Check sheet for the drawn part. Datum: minimum x, y, z corner. Units: mm. A direction names the side the tool comes from. Give positions to 0.01 mm unless a question says otherwise; leave off trailing zeros. Loops run counter-clockwise (first coordinate to the right, second up) from the corner with the lowest first, then second, coordinate; pieces in that order, holes last. Notation, with made-up numbers: (-28, 69.5) - (-22, 69.5) arc R26 ccw to (-22, 97.5) - close; hole circle Ø11 at (-34.75, 83.5). An arc over 180 degrees is marked (long way). Use one line per item in the form item = value.
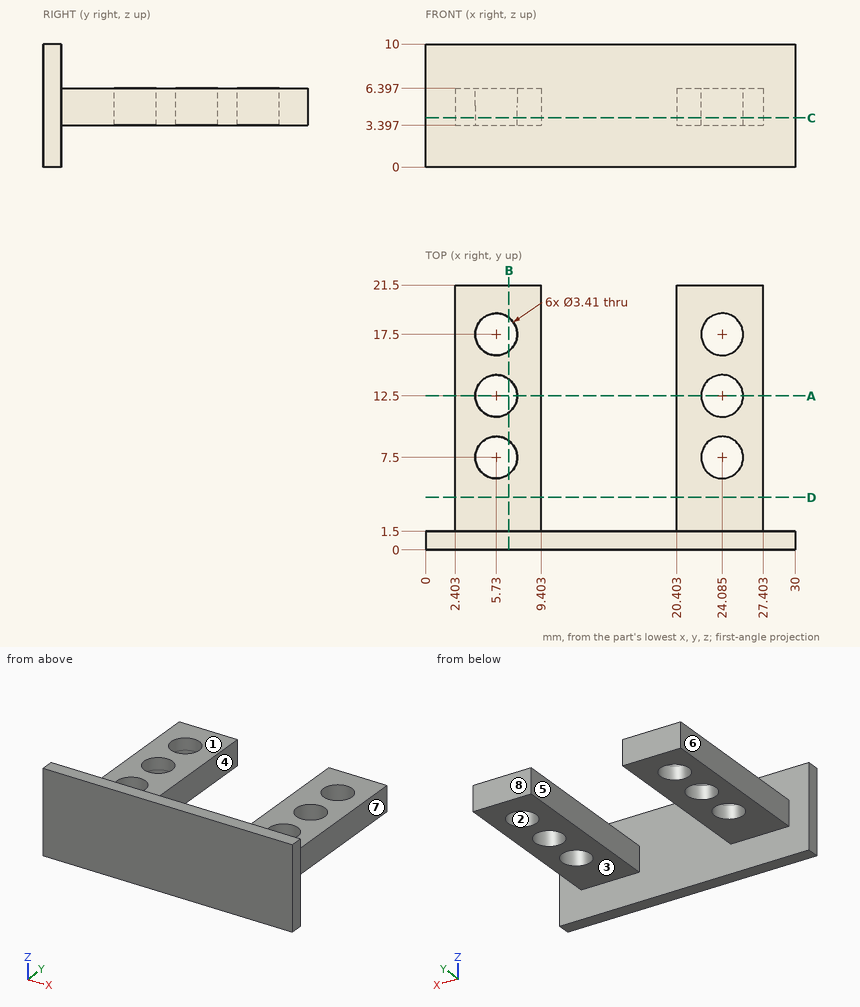
1. Scan lines: probe 1 along X at (y, z) = (12.5, 5.55) (1 decimal); probe 2 along X at (y, z) = (10.5, 4); probe 3 along Y at (x, z) = (10.25, 3.5). Record each from-to range of solid material in increasing order.
Result set:
probe_1 = 2.4 to 4, 7.4 to 9.4, 20.4 to 22.4, 25.8 to 27.4
probe_2 = 2.4 to 9.4, 20.4 to 27.4
probe_3 = 0 to 1.5
2. Section check D-D, the plane y = 4.25. Record the cut outline in (x, z), then the cut area to 3 significant figures.
Result set:
outline = (2.4, 3.4) - (9.4, 3.4) - (9.4, 6.4) - (2.4, 6.4) - close; (20.4, 3.4) - (27.4, 3.4) - (27.4, 6.4) - (20.4, 6.4) - close
area = 42.0 mm²
3. Section check A-A, the plane y = 12.5. Record the cut outline in (x, z) (1 decimal).
Result set:
outline = (2.4, 3.4) - (4, 3.4) - (4, 6.4) - (2.4, 6.4) - close; (7.4, 3.4) - (9.4, 3.4) - (9.4, 6.4) - (7.4, 6.4) - close; (20.4, 3.4) - (22.4, 3.4) - (22.4, 6.4) - (20.4, 6.4) - close; (25.8, 3.4) - (27.4, 3.4) - (27.4, 6.4) - (25.8, 6.4) - close
4. Section check B-B, the plane x = 6.75. Record the cut outline in (y, z).
Result set:
outline = (0, 0) - (1.5, 0) - (1.5, 3.4) - (6.13, 3.4) - (6.13, 6.4) - (1.5, 6.4) - (1.5, 10) - (0, 10) - close; (8.87, 3.4) - (11.13, 3.4) - (11.13, 6.4) - (8.87, 6.4) - close; (13.87, 3.4) - (16.13, 3.4) - (16.13, 6.4) - (13.87, 6.4) - close; (18.87, 3.4) - (21.5, 3.4) - (21.5, 6.4) - (18.87, 6.4) - close
5. Tool access check on the marked faces 1, 2, 3 and 4. Record the directions out of +Z, -Z, +X, -X, +Y, -Y that give a thin tool (end or side, any length) a straight path to the whole face; none if there is none.
Result set:
face_1 = +Z, +X, -X, +Y
face_2 = +Z, -Z
face_3 = -Z, +X, -X, +Y
face_4 = +Z, -Z, +Y
6. Draft check along X on the marked faces 5, 6, 7 and 8. Enter one of: released by +X, released by -X, zero draft, split by the parting line, or undercut.
Result set:
face_5 = undercut
face_6 = released by -X
face_7 = released by +X
face_8 = zero draft
7. Section check C-C, the plane z = 4. Record the cut outline in (x, y) (1 decimal).
Result set:
outline = (0, 0) - (30, 0) - (30, 1.5) - (27.4, 1.5) - (27.4, 21.5) - (20.4, 21.5) - (20.4, 1.5) - (9.4, 1.5) - (9.4, 21.5) - (2.4, 21.5) - (2.4, 1.5) - (0, 1.5) - close; hole circle Ø3.4 at (5.7, 7.5); hole circle Ø3.4 at (5.7, 12.5); hole circle Ø3.4 at (5.7, 17.5); hole circle Ø3.4 at (24.1, 7.5); hole circle Ø3.4 at (24.1, 12.5); hole circle Ø3.4 at (24.1, 17.5)
8. Depth check by flat-ended pin: pin 1 Ø4.5 at (x, y) = (24.08, 17.5) entering from +Z; pin 2 Ø3.5 at (y, z) = (9.5, 4.5) entering from +X; pin 3 Ø2 at (y, z) = (7, 4.5) entering from -X. Enter the tip coordinate at first touch or a pass-through.
Result set:
pin_1 = 6.4
pin_2 = 27.4
pin_3 = 2.4
